Here's how the part is built. I have some questions about the finished solid (model axes, mm). Face numbers are marked on the shaded views. Coordinates: 2 decimals unless noted, no trailing zeros. Write each loop counter-clockwise with the first axis right and the second up, starting at its lowest first coordinate (ties: lowest second). Pieces come first, ordered by that corner, then holes. Notation, with made-up numbers: (-30.5, 72.5) - (9.5, 72.5) arc R27 cw to (9.5, 104.5) - close; hole circle Ø8 at (-22, 2.25). An arc over 180 degrees is marked (long way). Answer in a Markdown table with one row per item. Add a question column.
Item 1: We'd pull the mould along Z, two halves only. Please class the marked faces 1, 2 and 3: +Z half, -Z half, draft (parallel to the pull), parting line (faces both ways), or undercut.
Item 2: Imagine slicing it at D-D (y = 24.5). Please give me the cut outline in (x, z), plus the area to 3 significant figures.
Item 3: Imagine slicing it at B-B (z = 0). Please give me the cut outline in (x, y).
Item 4: Imagine slicing it at A-A (x = 0). Please give me the cut outline in (y, z).
Item 5: If I drill on probe 1 along Z at (x, y) = (0, 6.5); probe 2 along Y at (x, z) = (-3.5, 0); probe 3 along X at (y, z) = (5.5, 0.5), over which ranges is the centre line in solid material (lowest first)? Write a range as from..to.
Item 6: Imagine slicing it at C-C (y = 17). Please give me the cut outline in (x, z), plus the area to 3 significant figures.
Item 7: I'm going to push flat-ended pins straight in: pin 1 (2.5 mm diameter, centred on y = 25, z = 0, fed in from -X); pin 2 (4 mm diameter, centred on y = 6, z = 2.5, fed in from +X); pin 3 (2 mm diameter, centred on y = 12, z = -3.5, fed in from +X). Where does each tip first touch, or does it pass through?
Autodesk Inventor part; units mm, degrees
ref_plane "YZ Plane" through (0, 0, 0) normal (1, 0, 0) x (0, 1, 0)
ref_plane "XZ Plane" through (0, 0, 0) normal (0, 1, 0) x (-1, 0, 0)
ref_plane "XY Plane" through (0, 0, 0) normal (0, 0, 1) x (1, 0, 0)
sketch "スケッチ1" plane through (0, 0, 0) normal (0, 1, 0) x (-1, 0, 0)
  circle A0 centre (0, 0) radius 6
  dimension "d0" = 12
extrude "押し出し1" add sketch "スケッチ1" along normal blind 30
sketch "スケッチ2" plane through (0, 0, 0) normal (0, -1, 0) x (1, 0, 0)
  circle A0 centre (0, 0) radius 2.5
  dimension "d3" = 5
extrude "押し出し2" cut sketch "スケッチ2" against normal blind 20
sketch "スケッチ3" plane through (0, 0, 0) normal (1, 0, 0) x (0, 1, 0)
  circle A0 centre (25, 0) radius 2
  line L0 (20, -2.5) -> (20, 2.5)
  point P0 (0, 0)
  dimension "d8" = 4
  dimension "d9" = 5
extrude "押し出し3" cut sketch "スケッチ3" along normal mid plane 20
properties part number "hand2_09"
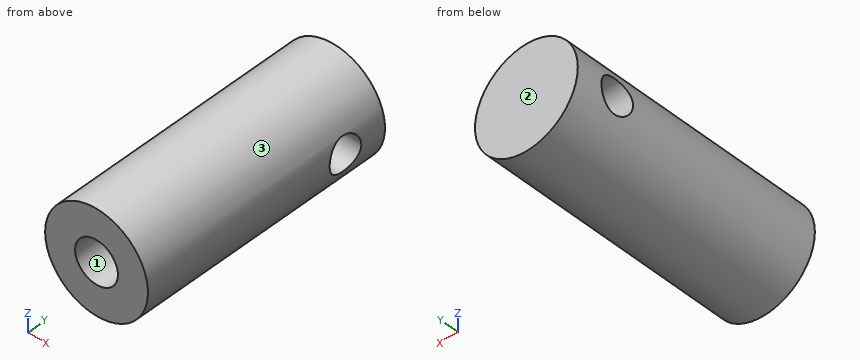
Here are the results:
| question | item | result |
|---|---|---|
| 1 | face 1 | undercut |
| 1 | face 2 | draft |
| 1 | face 3 | parting line |
| 2 | outline | (-5.68, -1.94) arc R6 ccw to (5.68, -1.94) - close; (-5.68, 1.94) - (5.68, 1.94) arc R6 ccw to start |
| 2 | area | 67.4 mm2 |
| 3 | outline | (-6, 0) - (-2.5, 0) - (-2.5, 20) - (2.5, 20) - (2.5, 0) - (6, 0) - (6, 23) - (-6, 23) - close; (-6, 27) - (6, 27) - (6, 30) - (-6, 30) - close |
| 4 | outline | (0, -6) - (30, -6) - (30, 6) - (0, 6) - (0, 2.5) - (20, 2.5) - (20, -2.5) - (0, -2.5) - close; hole circle Ø4 at (25, 0) |
| 5 | probe 1 | z = -6..-2.5, 2.5..6 |
| 5 | probe 2 | y = 0..23, 27..30 |
| 5 | probe 3 | x = -5.98..-2.45, 2.45..5.98 |
| 6 | outline | circle Ø12 at (0, 0); hole circle Ø5 at (0, 0) |
| 6 | area | 93.5 mm2 |
| 7 | pin 1 | passes through |
| 7 | pin 2 | stops at x = 5.98 |
| 7 | pin 3 | stops at x = 5.45 |
